Source: CAD feature listing. Evaluate the final solid. Frame: model axes, mm. Face numbers are marked on the shaded views. A direction names the side the tool comes from. Coordinates: 2 decimals unless noted, no trailing zeros. Write each loop counter-clockwise with the first axis right and the second up, starting at its lowest first coordinate (ties: lowest second). Pieces come first, ordered by that corner, then holes. Notation, with made-up numbers: (-32, 43.25) - (-25, 43.25) arc R21 cw to (-25, 51.25) - close; hole circle Ø6 at (24.5, 67). An arc over 180 degrees is marked (long way). One line per question, with ' | ' between items.
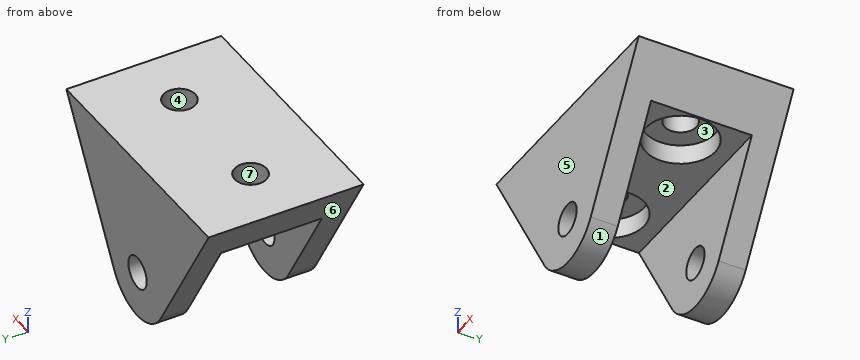
from build123d import *

# Parameters (mm, degrees)
BOSS_EXTRUDE1_DEPTH                                  = 50.8
CBORE_FOR_1_4_BINDING_HEAD_MACHINE_SCREW_D           = 6.5278
CBORE_FOR_1_4_BINDING_HEAD_MACHINE_SCREW_CBORE_D     = 14.2875
CBORE_FOR_1_4_BINDING_HEAD_MACHINE_SCREW_CBORE_DEPTH = 4.064
CUT_EXTRUDE1_REACH                                   = 75.909
SKETCH4_R                                            = 3.2639


with BuildPart() as part:
    # Sketch1 → Boss-Extrude1 (new body)
    with BuildSketch(Plane(origin=(0, 0, 0), x_dir=(0, 0, -1), z_dir=(1, 0, 0))):
        Polygon((0, 0), (0, 31.75), (43.28806111, 31.75), (43.28806111, 26.2001), (8.89, 26.2001), (8.89, 5.5499), (43.28806111, 5.5499), (43.28806111, 0), align=None)
    extrude(amount=BOSS_EXTRUDE1_DEPTH)

    # CBORE for 1/4 Binding Head Machine Screw1 (through all)
    with Locations(Plane(origin=(0, 0, -8.89), x_dir=(-1, 0, 0), z_dir=(0, 0, -1))):
        with Locations((-12.7, 15.875), (-38.1, 15.875)):
            CounterBoreHole(CBORE_FOR_1_4_BINDING_HEAD_MACHINE_SCREW_D / 2, CBORE_FOR_1_4_BINDING_HEAD_MACHINE_SCREW_CBORE_D / 2, CBORE_FOR_1_4_BINDING_HEAD_MACHINE_SCREW_CBORE_DEPTH)

    # Cut-Extrude1: up to this face of the body (flat: up to its plane)
    cut_extrude1_end = Plane(part.part.faces().sort_by_distance((25.4, 31.75, -21.644030555))[0])
    # Sketch4 → Cut-Extrude1 (cut, up to the picked face)
    with BuildSketch(Plane.XZ, mode=Mode.PRIVATE) as cut_extrude1_sk1:
        with Locations(Location((25.4, -24.188970368, 0), (0, 0, 270))):
            Circle(SKETCH4_R)
    cut_extrude1_tool1 = split(extrude(cut_extrude1_sk1.sketch, amount=-CUT_EXTRUDE1_REACH, mode=Mode.PRIVATE), bisect_by=cut_extrude1_end, keep=Keep.BOTH, mode=Mode.PRIVATE)
    # Sketch4 → Cut-Extrude1 (cut, up to the picked face)
    with BuildSketch(Plane.XZ, mode=Mode.PRIVATE) as cut_extrude1_sk2:
        with BuildLine():
            Line((17.115609678, -29.067079653), (0, 0))
            Line((0, 0), (0, -43.28806111))
            Line((0, -43.28806111), (50.8, -43.28806111))
            Line((50.8, -43.28806111), (50.8, 0))
            Line((50.8, 0), (33.684390322, -29.067079653))
            ThreePointArc((33.684390322, -29.067079653), (25.4, -33.802870368), (17.115609678, -29.067079653))
        make_face()
    cut_extrude1_tool2 = split(extrude(cut_extrude1_sk2.sketch, amount=-CUT_EXTRUDE1_REACH, mode=Mode.PRIVATE), bisect_by=cut_extrude1_end, keep=Keep.BOTH, mode=Mode.PRIVATE)
    add(cut_extrude1_tool1.solids().sort_by(Axis((25.4, 0, -24.18897), (0, 1, 0)))[0], mode=Mode.SUBTRACT)
    add(cut_extrude1_tool2.solids().sort_by(Axis((7.982682, 0, -14.87219), (0, 1, 0)))[0], mode=Mode.SUBTRACT)


solid = part.part
Item 1: Ray query, line 1 along Y through (x, z) = (14, -17); line 2 along X through (y, z) = (17, -4); line 3 along Y through (x, z) = (38.1, -6.75). Return the intervals inside material, ascending. Write a range as [from, to].
Check sheet entries:
line 1: [0, 5.55], [26.2, 31.75] | line 2: [2.36, 9.64], [15.76, 35.04], [41.16, 48.44] | line 3: [0, 8.73], [23.02, 31.75]
Item 2: Cut plane C-C on x = 15. Return loops of the section in (y, z), and give its area (3 significant figures).
Check sheet entries:
outline: (0, -25.47) - (5.55, -25.47) - (5.55, -8.89) - (9.11, -8.89) - (9.11, -4.83) - (13.56, -4.83) - (13.56, 0) - (0, 0) - close; (18.19, -4.83) - (22.64, -4.83) - (22.64, -8.89) - (26.2, -8.89) - (26.2, -25.47) - (31.75, -25.47) - (31.75, 0) - (18.19, 0) - close | area: 389 mm²
Item 3: Pin query (flat end, axial travel): pin 1 Ø11.5 at (x, y) = (12.7, 15.875) entering from +Z; pin 2 Ø10.5 at (x, y) = (28, 16.5) entering from -Z; pin 3 Ø1 at (y, z) = (18, -6.5) entering from +X; pin 4 Ø7.5 at (x, y) = (38.1, 15.875) entering from -Z. Return the tip coordinate at first contact, or that it passes through.
Check sheet entries:
pin 1: z = 0 | pin 2: z = -8.89 | pin 3: x = 47.27 | pin 4: z = -4.83
Item 4: Mould query, pull axis Y, two halves, no side actions, for the marked faces 4, 5, 6 and 7. Classes: pulls with the +Y half, pulls with the -Y half, needs draft (parallel to the pull), parting line crosses it, or undercut.
Check sheet entries:
face 4: undercut | face 5: pulls with the -Y half | face 6: needs draft | face 7: undercut
Item 5: Cut plane B-B on z = -30. Return loops of the section in (x, y).
Check sheet entries:
outline: (17.74, 0) - (33.06, 0) - (33.06, 5.55) - (17.74, 5.55) - close; (17.74, 26.2) - (33.06, 26.2) - (33.06, 31.75) - (17.74, 31.75) - close
Item 6: Access query for the marked faces 1, 2 and 3. Directions: +Z, -Z, +X, -X, +Y, -Y. A direction counts if a zero-diameter tool reaches every point of the face in a straight line with its end or side. Return the directions, or none.
Check sheet entries:
face 1: -Z, +Y, -Y | face 2: -Z, +X, -X | face 3: -Z
Item 7: Cut plane D-D on z = -26. Return loops of the section in (x, y), and give its area (3 significant figures).
Check sheet entries:
outline: (15.31, 0) - (22.68, 0) - (22.68, 5.55) - (15.31, 5.55) - close; (15.31, 26.2) - (22.68, 26.2) - (22.68, 31.75) - (15.31, 31.75) - close; (28.12, 0) - (35.49, 0) - (35.49, 5.55) - (28.12, 5.55) - close; (28.12, 26.2) - (35.49, 26.2) - (35.49, 31.75) - (28.12, 31.75) - close | area: 164 mm²
Item 8: Cut plane A-A on x = 25.4. Return loops of the section in (y, z).
Check sheet entries:
outline: (0, -33.8) - (5.55, -33.8) - (5.55, -27.45) - (0, -27.45) - close; (0, -20.93) - (5.55, -20.93) - (5.55, -8.89) - (26.2, -8.89) - (26.2, -20.93) - (31.75, -20.93) - (31.75, 0) - (0, 0) - close; (26.2, -33.8) - (31.75, -33.8) - (31.75, -27.45) - (26.2, -27.45) - close
